from build123d import *

# Parameters (mm, degrees)
SKETCH1_R           = 3
BOSS_EXTRUDE1_DEPTH = 10


with BuildPart() as part:
    # Sketch1 → Boss-Extrude1 (new body)
    with BuildSketch(Plane.XY):
        with BuildLine():
            Line((10.5, 0), (0, 0))
            Line((0, 0), (-1.022323327, 1.510963722))
            Line((-1.022323327, 1.510963722), (-0.603635677, 9.5))
            ThreePointArc((-0.603635677, 9.5), (-6.462853921, 8.095985117), (-11.9, 5.5))
            Line((-11.9, 5.5), (-9.686017962, 4.221756874))
            Line((-9.686017962, 4.221756874), (-10.9, -0.318754948))
            Line((-10.9, -0.318754948), (-11.9, -0.318754948))
            Line((-11.9, -0.318754948), (-11.9, -2.769258551))
            ThreePointArc((-11.9, -2.769258551), (-10.648945281, -6.93734622), (-6.81703295, -9))
            Line((-6.81703295, -9), (-6.81703295, -6))
            Line((-6.81703295, -6), (-4.81703295, -6))
            Line((-4.81703295, -6), (-4.81703295, -9))
            add(Edge.make_bspline(
                [(-4.81703295, -9), (2.115225064, -8.331257602), (12.97604793, -9.010983468), (15.5, 0)],
                knots=[0.063235072, 0.063235072, 0.063235072, 0.063235072, 1.063235072, 1.063235072, 1.063235072, 1.063235072], degree=3))
            ThreePointArc((15.5, 0), (13, 2.5), (10.5, 0))
        make_face()
        with Locations((-6.8, 0)):
            Circle(SKETCH1_R, mode=Mode.SUBTRACT)
    extrude(amount=BOSS_EXTRUDE1_DEPTH)


solid = part.part
Geometry check sheet. Reference: the model listing, model coordinates, mm. A direction names the side the tool comes from. Give positions to 0.01 mm unless a question says otherwise; leave off trailing zeros. Loops run counter-clockwise (first coordinate to the right, second up) from the corner with the lowest first, then second, coordinate; pieces in that order, holes last. Notation, with made-up numbers: M 28,59 L 44,59 A25 ccw 44,83 Z; hole C -8,33 d7. An arc over 180 degrees is marked long. Write each question's results on one line, items separated by ' | '.
1) Gauge pin test, flat ends, axial feed: pin 1 (1 mm diameter, centred on x = -5.5, z = 5.5, fed in from -Y); pin 2 (2 mm diameter, centred on y = -1, z = 6, fed in from -X); pin 3 (1.5 mm diameter, centred on y = -7, z = 4, fed in from +X). Record the tip position at first contact, or that the pin passes through.
Answers follow:
pin 1: y = -6 | pin 2: x = -11.9 | pin 3: x = 10.54
2) Release check for a two-part mould opening along Y. For faces 4 (the face through (-10.285, 1.983, 4.93)), 5 (the face through (-6.817, -8, 5)), 6 (the face through (13.1, 2.5, 4.9)) record: +Y half, -Y half, draft (parallel to the pull), parting line (faces both ways), or undercut.
Answers follow:
face 4: undercut | face 5: draft | face 6: +Y half
3) Section check B-B, the plane y = 7. Record the boundary of the cut face in (x, z), plus the area to 3 significant figures.
Answers follow:
outline: M -9.13,0 L -0.73,0 L -0.73,10 L -9.13,10 Z | area: 83.9 mm2
4) Thickness scan on line 1 (X direction, y = 0.5, z = 8.25); line 2 (Y direction, x = -6.5, z = 5.75); line 3 (Y direction, x = -1.5, z = 9.25). Record the ranges inside material, lowest first.
Answers follow:
line 1: -10.68 to -9.76, -3.84 to -0.34, 10.55 to 15.45 | line 2: -6 to -2.98, 2.98 to 8.08 | line 3: -8.75 to 9.37
5) Tool access check on faces 1 (the face through (-10.81, 4.87, 4.93)), 2 (the face through (5, 0, 5)), 3 (the face through (-0.5, 0.74, 4.93)). Record the directions out of +Z, -Z, +X, -X, +Y, -Y that give a thin tool (end or side, any length) a straight path to the whole face; none if there is none.
Answers follow:
face 1: +Z, -Z, -X | face 2: +Z, -Z, +Y | face 3: +Z, -Z
6) Section check A-A, the plane x = -6.5. Record the boundary of the cut face in (y, z).
Answers follow:
outline: M -6,0 L -2.98,0 L -2.98,10 L -6,10 Z; M 2.98,0 L 8.08,0 L 8.08,10 L 2.98,10 Z
